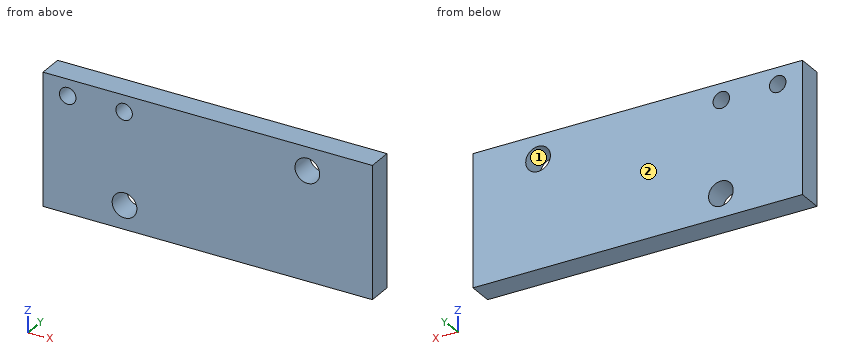
```python
from build123d import *

# Parameters (mm, degrees)
SKETCH1_W           = 40
SKETCH1_H           = 16
SKETCH1_R           = 1.5
BOSS_EXTRUDE1_DEPTH = 3
SKETCH2_R           = 1
CUT_EXTRUDE1_DEPTH  = 10


with BuildPart() as part:
    # Sketch1 → Boss-Extrude1 (new body)
    with BuildSketch(Plane(origin=(0, 0, 0), x_dir=(1, 0, 0), z_dir=(0, 1, 0))):
        with Locations((20, 8)):
            Rectangle(SKETCH1_W, SKETCH1_H)
        with Locations((9.9, 13.13)):
            Circle(SKETCH1_R, mode=Mode.SUBTRACT)
        with Locations((32.1, 2.83)):
            Circle(SKETCH1_R, mode=Mode.SUBTRACT)
    extrude(amount=BOSS_EXTRUDE1_DEPTH)

    # Sketch2 → Cut-Extrude1 (cut)
    with BuildSketch(Plane(origin=(0, 3, 0), x_dir=(1, 0, 0), z_dir=(0, 1, 0))):
        with Locations((3, 2)):
            Circle(SKETCH2_R)
        with Locations((9.85, 2)):
            Circle(SKETCH2_R)
    extrude(amount=-CUT_EXTRUDE1_DEPTH, mode=Mode.SUBTRACT)


solid = part.part
```
Build history of the part. All positions in model axes, mm. Face numbers are marked on the shaded views. Give positions to 0.01 mm unless a question says otherwise; leave off trailing zeros. Order: outer loops, then holes, each group sorted by start corner. A loop starts at its lowest first (then second) coordinate and runs counter-clockwise, first axis right, second up. Notation, with made-up numbers: M -23.75,74 L 4.25,74 A17 cw 4.25,97 Z; hole C 28,49.5 d2. An arc over 180 degrees is marked long. Write item = value, one per line. Start each with the question number.
(1) Slice it at A-A on x = 3. Write the cut outline in (y, z).
(2) Slice it at B-B on y = 0.6. Write the cut outline in (x, z).
(3) Pin check, flat tip, straight feed: pin 1 Ø1.6 at (x, z) = (3, -2) entering from -Y. Stop position of the tip, or through.
(4) Slice it at D-D on x = 9.9. Write the cut outline in (y, z).
(5) Slice it at C-C on z = -13.13. Write the cut outline in (x, y).
(6) Two-plate mould, pull along X, no slides. Class the marked faces 1 and 2: released by +X, released by -X, zero draft, split by the parting line, or undercut.
(7) Probe L1, parallel to X at y = 1.8, z = -13.13; L2, parallel to X at y = 1.25, z = -2; L3, parallel to X at y = 1.65, z = -2.83. List the from-to ranges inside material, lowest first. Write a range as [from, to].
Responses:
q1.outline = M 0,-16 L 3,-16 L 3,-3 L 0,-3 Z; M 0,-1 L 3,-1 L 3,0 L 0,0 Z
q2.outline = M 0,-16 L 40,-16 L 40,0 L 0,0 Z; hole C 3,-2 d2; hole C 9.9,-13.13 d3; hole C 9.85,-2 d2; hole C 32.1,-2.83 d3
q3.pin_1 = through
q4.outline = M 0,-16 L 3,-16 L 3,-14.63 L 0,-14.63 Z; M 0,-11.63 L 3,-11.63 L 3,-3 L 0,-3 Z; M 0,-1 L 3,-1 L 3,0 L 0,0 Z
q5.outline = M 0,0 L 8.4,0 L 8.4,3 L 0,3 Z; M 11.4,0 L 40,0 L 40,3 L 11.4,3 Z
q6.face_1 = undercut
q6.face_2 = zero draft
q7.L1 = [0, 8.4], [11.4, 40]
q7.L2 = [0, 2], [4, 8.85], [10.85, 30.85], [33.35, 40]
q7.L3 = [0, 2.44], [3.56, 9.29], [10.41, 30.6], [33.6, 40]
